Work out the finished part from the listing and answer in its coordinate system (mm). Face numbers are marked on the shaded views. A direction names the side the tool comes from. Coordinates: 2 decimals unless noted, no trailing zeros. Order: outer loops, then holes, each group sorted by start corner. A loop starts at its lowest first (then second) coordinate and runs counter-clockwise, first axis right, second up. Notation, with made-up numbers: (-17.75, 78.25) -> (20.25, 78.25) arc R11 ccw to (20.25, 99.25) -> close; hole circle Ø4 at (55, 61). An arc over 180 degrees is marked (long way). Answer as CSV lines item,"result". Start each with the question number.
Item 1: Which of the six approach directions +Z, -Z, +X, -X, +Y, -Y give full straight-line access (tool end or side, diameter ignored) to the marked faces 5 and 6?
Item 2: Straight lines are drawn through the part: L1, parallel to Y at x = -3, z = 54; L2, parallel to Z at x = 46, y = 12; L3, parallel to Z at x = -40, y = -55. For each, find the intervals that lie inside material, in ascending order.
Item 3: Section B-B (y = -7.5) is taken. Write down the section's boundary in (x, z), then the cut area to 3 significant figures.
Item 4: Section A-A (z = 59) is taken. Write down the section's boundary in (x, y).
Item 5: Section C-C (x = -72) is taken. Write down the section's boundary in (y, z), then the cut area to 3 significant figures.
Item 6: Section D-D (y = 57.5) is taken. Write down the section's boundary in (x, z).
Item 7: For a pull along X with two mould halves and no side action, classify the marked faces 1, 2, 3 and 4 as pulls with the +X half, pulls with the -X half, needs draft (parallel to the pull), parting line crosses it, or undercut.
Item 8: Each of these flat-tipped pins is pushed along its axis until it touches: pin 1 Ø5 at (x, y) = (13, -8.5) entering from +Z; pin 2 Ø12 at (x, y) = (-17, -9.5) entering from +Z; pin 3 Ø3 at (x, z) = (23.5, 79.5) entering from -Y. Where does it stop, or does it pass through?
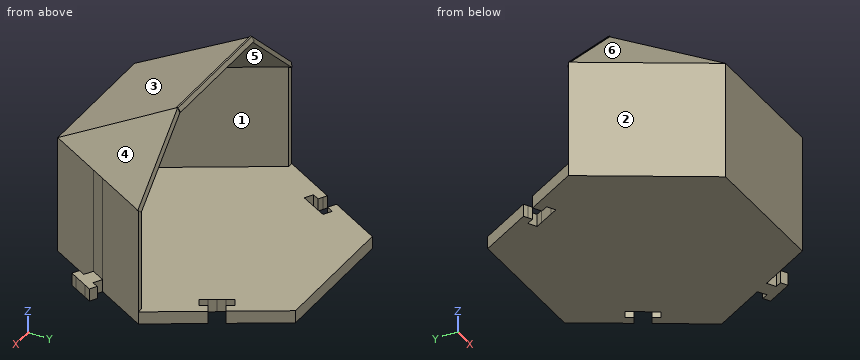
```python
from build123d import *

# Parameters (mm, degrees)
F0_W      = 50
F0_H      = 12.5
F1_DEPTH  = 8
F2_DEPTH  = 75
F4_DEPTH  = 8
F7_DEPTH  = 3
F8_DEPTH  = 1
F11_DEPTH = 3
F14_DEPTH = 3
F15_DEPTH = 8
F16_DEPTH = 8
F17_DEPTH = 8
F18_DEPTH = 8


# Not quite as in the source:
# - a feature names something its author has since deleted; it is built from what else it names


with BuildPart() as f1:
    # F0 (on Top) → F1 (new body)
    with BuildSketch(Plane.XY):
        Polygon((-42.0179491924, 72.7772228311), (-60.5095952989, 40.7487522591), (-57.9695070384, 39.3207329262), (-55.5194165334, 43.6791064608), (-50.2642610162, 40.7248836223), (-52.7144317239, 36.366367418), (-57.615009792, 27.6494680496), (-60.0654171506, 23.2910848888), (-65.3204122546, 26.2455930623), (-62.870004896, 30.6039762231), (-65.5097997054, 32.0881441788), (-84.0358983849, 0), (-42.0179491924, -72.7772228311), (42.0179491924, -72.7772228311), (84.0358983849, 0), (65.5097997054, 32.0881441788), (62.870004896, 30.6039762231), (65.3204122546, 26.2455930623), (60.0654171506, 23.2910848888), (57.615009792, 27.6494680496), (55.164720758, 32.0079177338), (52.7144317239, 36.366367418), (50.2642610162, 40.7248836223), (55.5194165334, 43.6791064608), (57.9695070384, 39.3207329262), (60.5095952989, 40.7487522591), (42.0179491924, 72.7772228311), align=None)
        with Locations((0, 54.5829171234)):
            Rectangle(F0_W, F0_H, mode=Mode.SUBTRACT)
    extrude(amount=F1_DEPTH)

    # F0 (on Top) → F2 (join)
    with BuildSketch(Plane.XY):
        Polygon((68.1424599038, -33.5282429562), (87.5, 0), (84.0358983849, 0), (42.0179491924, -72.7772228311), (-42.0179491924, -72.7772228311), (-84.0358983849, 0), (-87.5, 0), (-43.75, -75.7772228311), (43.75, -75.7772228311), (63.1424599038, -42.188496994), align=None)
    extrude(amount=F2_DEPTH)

    # F0 (on Top) → F4 (join)
    with BuildSketch(Plane.XY):
        Polygon((43.75, 75.7772228311), (-43.75, 75.7772228311), (-63.1248363216, 42.2190219338), (-60.5095952989, 40.7487522591), (-42.0179491924, 72.7772228311), (42.0179491924, 72.7772228311), (60.5095952989, 40.7487522591), (63.1248363216, 42.2190219338), align=None)
    extrude(amount=F4_DEPTH)

    # F6 (on face) → F7 (join)
    with BuildSketch(Plane(origin=(0, -50.1312366318, 89.3836679776), x_dir=(1, 0, 0), z_dir=(0, 0.4891706574, -0.872188092))):
        Polygon((43.75, 29.4041920927), (0, 29.4041920927), (-43.75, 29.4041920927), (-42.01795, -57.4775522498), (42.01795, -57.4775522498), align=None)
    extrude(amount=F7_DEPTH)

    # F3 (on Front) → F8 (join)
    with BuildSketch(Plane.XZ):
        Polygon((-42.01795, 114.5), (0, 114.5), (42.01795, 114.5), (84.0359, 75), (87.5, 75), (42.01795, 117.5), (0, 117.5), (-42.01795, 117.5), (-87.5, 75), (-84.0359, 75), align=None)
    extrude(amount=F8_DEPTH)

    # F10 (on face) → F11 (join)
    with BuildSketch(Plane(origin=(-67.6846727043, -39.0777640058, 72.4338274863), x_dir=(0.7723629594, -0.3015876344, 0.5590173143), z_dir=(-0.6351814378, -0.3667221741, 0.6797495039))):
        Polygon((33.2314262259, 55.789645187), (-25.6554603702, 35.6104118215), (30.9888924807, -31.0804218073), align=None)
    extrude(amount=-F11_DEPTH)

    # F13 (on face) → F14 (join)
    with BuildSketch(Plane(origin=(67.6756688636, -39.5950852503, 72.4241918832), x_dir=(0.7733047167, 0.3041472681, -0.556322078), z_dir=(-0.6340345536, 0.3709553614, -0.6785221475))):
        Polygon((-30.939509805, 30.5117392321), (-32.8751652468, -56.3649154418), (25.9400068576, -35.9776056011), align=None)
    extrude(amount=F14_DEPTH)

    # F0 (on Top) → F15 (join)
    with BuildSketch(Plane.XY):
        with Locations((0, 54.5829171234)):
            Rectangle(F0_W, F0_H)
    extrude(amount=F15_DEPTH)

    # F0 (on Top) → F16 (join)
    with BuildSketch(Plane.XY):
        Polygon((75.7376143812, -32.7192219692), (73.5984199476, -36.6782429562), (77.9285469666, -39.1782429562), (80.1153549422, -35.2453215385), align=None)
        Polygon((73.5984199476, -36.6782429562), (68.1424599038, -33.5282429562), (63.1424599038, -42.188496994), (68.5982950526, -45.3387133087), (72.9283229484, -47.838884987), (77.9285469666, -39.1782429562), align=None)
        Polygon((72.9283229484, -47.838884987), (68.5982950526, -45.3387133087), (66.3481405421, -49.235738415), (70.6781684379, -51.7359100933), align=None)
    extrude(amount=F16_DEPTH)

    # F0 (on Top) → F17 (join)
    with BuildSketch(Plane.XY):
        Polygon((-65.5097997054, 32.0881441788), (-68.125, 33.5584843966), (-87.5, 0), (-84.0358983849, 0), align=None)
    extrude(amount=F17_DEPTH)

    # F0 (on Top) → F18 (join)
    with BuildSketch(Plane.XY):
        Polygon((87.5, 0), (68.125, 33.5584843966), (65.5097997054, 32.0881441788), (84.0358983849, 0), align=None)
    extrude(amount=F18_DEPTH)


solid = f1.part
```
Checked values:
1,face 5,"+Y"
1,face 6,"+Z, -X, -Y"
2,L1,"y = -75.78 to -72.78"
2,L2,"z = 0 to 8"
2,L3,"z = 0 to 8, 83.21 to 86.65"
3,outline,"(-83.17, 0) -> (83.17, 0) -> (83.17, 75) -> (83.45, 75.23) -> (42.4, 113.59) -> (42.19, 113.29) -> (-42.19, 113.29) -> (-83.17, 75) -> close; hole (-79.71, 8) -> (79.71, 8) -> (79.71, 74.31) -> (41.67, 109.85) -> (-41.15, 109.85) -> (-79.71, 73.82) -> close"
3,area,"2,430 mm^2"
4,outline,"(-87.5, 0) -> (-43.75, -75.78) -> (43.75, -75.78) -> (87.5, 0) -> (84.04, 0) -> (42.02, -72.78) -> (-42.02, -72.78) -> (-84.04, 0) -> close"
5,outline,"(-26.85, 0) -> (26.85, 0) -> (26.85, 8) -> (-20.85, 8) -> (-20.85, 73.82) -> (1.1, 85.66) -> (0, 89.48) -> (-1, 89.48) -> (-1, 88.94) -> (-26.85, 75) -> close"
5,area,"936 mm^2"
6,outline,"(-54.3, 0) -> (54.3, 0) -> (54.3, 8) -> (-54.3, 8) -> close"
7,face 1,"undercut"
7,face 2,"pulls with the -X half"
7,face 3,"needs draft"
7,face 4,"pulls with the +X half"
8,pin 1,"stops at z = 114.13"
8,pin 2,"stops at z = 115.54"
8,pin 3,"stops at y = -70.43"
